from build123d import *

# Parameters (mm, degrees)
ESQUISSE2_R                  = 3
ENL_V_MAT_EXTRU_1_DEPTH      = 3
ESQUISSE3_R                  = 1.75
ENL_V_MAT_EXTRU_2_DEPTH      = 4
ENL_V_MAT_EXTRU_2_DEPTH_BACK = 13


with BuildPart() as part:
    # Esquisse1 → Révolution1 (revolve)
    with BuildSketch(Plane.XY):
        Polygon((-7.5, 0), (7.5, 0), (7.5, 12), (7, 12), (5, 8), (-5, 8), (-7, 12), (-7.5, 12), align=None)
    revolve(axis=Axis((0, 0, 0), (-1, 0, 0)))

    # Esquisse2 → Enlèv. mat.-Extru.1 (cut)
    with BuildSketch(Plane(origin=(7.5, 0, 0), x_dir=(0, 0, -1), z_dir=(1, 0, 0))):
        Circle(ESQUISSE2_R)
    extrude(amount=-ENL_V_MAT_EXTRU_1_DEPTH, mode=Mode.SUBTRACT)

    # Esquisse3 → Enlèv. mat.-Extru.2 (cut, two sides)
    with BuildSketch(Plane(origin=(4.5, 0, 0), x_dir=(0, 0, -1), z_dir=(1, 0, 0))) as enl_v_mat_extru_2_sk:
        Circle(ESQUISSE3_R)
    extrude(amount=ENL_V_MAT_EXTRU_2_DEPTH, mode=Mode.SUBTRACT)
    extrude(enl_v_mat_extru_2_sk.sketch, amount=-ENL_V_MAT_EXTRU_2_DEPTH_BACK, mode=Mode.SUBTRACT)


solid = part.part
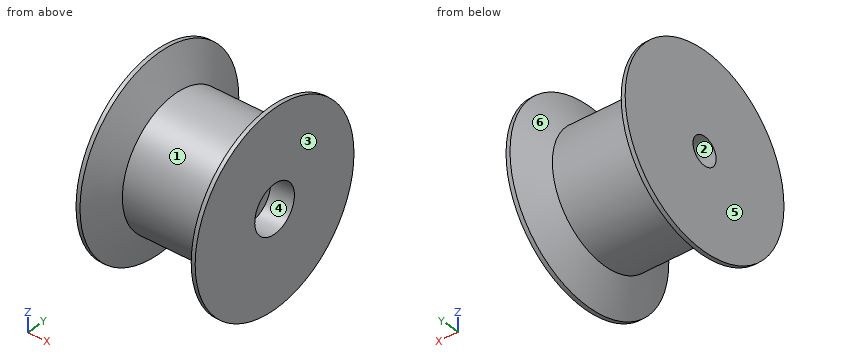
The listing builds one solid part. Answer for the finished solid, in the listing's coordinates (mm). Face numbers are marked on the shaded views. A direction names the side the tool comes from. Coordinates: 2 decimals unless noted, no trailing zeros. Loops run counter-clockwise (first coordinate to the right, second up) from the corner with the lowest first, then second, coordinate; pieces in that order, holes last.
1) Find the intervals of material crossed by L1, parallel to Y at x = 0.25, z = 0; L2, parallel to X at y = -2.5, z = -1.5; L3, parallel to X at y = -1, z = 11, in increasing order.
2) Find section A-A on y = 0. Write down the section's boundary in (x, z).
3) Flat-ended cylindrical pins translate along their axes: pin 1 Ø1 at (x, z) = (1, 6) entering from -Y; pin 2 Ø1 at (x, y) = (4, 7) entering from -Z; pin 3 Ø3 at (x, z) = (5.5, -6) entering from +Y. Find the tip coordinate at first contact, or state that the pin passes through.
4) A tool of negligible diameter and unlimited length cuts with its end or side. For the marked faces 4, 5 and 6, from which of +Z, -Z, +X, -X, +Y, -Y can it reach the whole face along a straight path? Write none if from no direction.
5) Find section C-C on x = -5.5. Write down the section's boundary in (y, z), then the cut area to 3 significant figures.
6) Determine the mould class of the marked faces 1, 2 and 3 for opening direction Z: pulls with the +Z half, pulls with the -Z half, needs draft (parallel to the pull), parting line crosses it, or undercut.
Values:
1. L1: y = -8 to -1.75, 1.75 to 8
1. L2: x = -7.5 to 4.5
1. L3: x = -7.5 to -6.52, 6.52 to 7.5
2. outline: (-7.5, -12) - (-7, -12) - (-5, -8) - (5, -8) - (7, -12) - (7.5, -12) - (7.5, -3) - (4.5, -3) - (4.5, -1.75) - (-7.5, -1.75) - close; (-7.5, 1.75) - (4.5, 1.75) - (4.5, 3) - (7.5, 3) - (7.5, 12) - (7, 12) - (5, 8) - (-5, 8) - (-7, 12) - (-7.5, 12) - close
3. pin 1: stops at y = -5.81
3. pin 2: stops at z = -4.66
3. pin 3: stops at y = 10.49
4. face 4: +X
4. face 5: +Z, -Z, -X, +Y, -Y
4. face 6: none
5. outline: circle Ø18 at (0, 0); hole circle Ø3.5 at (0, 0)
5. area: 245 mm2
6. face 1: parting line crosses it
6. face 2: undercut
6. face 3: needs draft
